The model under review builds one solid part; all positions refer to its coordinate system, in mm. A direction names the side the tool comes from. Round coordinates to 2 decimals unless told otherwise and drop trailing zeros. Write each loop counter-clockwise with the first axis right and the second up, starting at its lowest first coordinate (ties: lowest second). Pieces come first, ordered by that corner, then holes. Notation, with made-up numbers: (31, 69.5) -> (57, 69.5) arc R24 cw to (57, 84.5) -> close; hole circle Ø11 at (38.25, -35). An arc over 180 degrees is marked (long way). Use CSV: the item, a comma, the result in double quotes. Start each with the question number.
1) Take a section at C-C, the plane z = 3.5. Give the boundary of the cut face in (x, y).
2) Mouldability with a two-part tool opening along X and no side actions: class faces 4 (the face through (21.4, -0.1, 0.5)), 5 (the face through (-21.4, -0.1, 0.5)), 6 (the face through (-13, -0.76, 6.28)), 7 (the face through (-20.45, 8.5, 0.51)) as released by +X, released by -X, zero draft, split by the parting line, or undercut.
3) Take a section at B-B, the plane x = 15.4. Give the boundary of the cut face in (y, z), then the cut area to 3 significant figures.
4) Take a section at A-A, the plane y = 7.5. Give the boundary of the cut face in (x, z).
5) Machinability: for faces 1 (the face through (11.7, 7, 6)), 2 (the face through (0.55, -3, 6)), 3 (the face through (7, 5.25, 6)), which of the approach directions +Z, -Z, +X, -X, +Y, -Y give a long, thin tool a straight path to every point of the face, cutting with its end or side? Answer none if there is none.
6) For pin 1 Ø4.5 at (y, z) = (8.5, 6.5) entering from +X; pin 2 Ø3 at (y, z) = (-7.5, 8) entering from +X; pin 3 Ø5.5 at (x, z) = (3.5, 5.5) entering from -Y; pin 4 Ø2.5 at (x, y) = (15.4, -8.5) entering from +Z, all flat-tipped, find the tip position at first contact; note any pin that passes through.
7) Wall thickness on probe 1 along Y at (x, z) = (-20.05, 0.25); probe 2 along Y at (x, z) = (8.5, 10.25); probe 3 along Z at (x, y) = (-19, 8): over which ranges is each line inside the solid? List them lowest first. Write a range as [from, to].
8) Take a section at D-D, the plane y = 0.75. Give the boundary of the cut face in (x, z).
from build123d import *

# Parameters (mm, degrees)
SKETCH1_W           = 42.8
SKETCH1_H           = 20.5
SKETCH1_R           = 1.4
BOSS_EXTRUDE1_DEPTH = 1
SKETCH3_R           = 3.95
SKETCH3_W           = 9.3
SKETCH3_H           = 4.3
SKETCH3_W_2         = 12.05
SKETCH3_H_2         = 12.05
BOSS_EXTRUDE2_DEPTH = 10.7
SKETCH4_R           = 0.5
CUT_EXTRUDE1_DEPTH  = 2


with BuildPart() as part:
    # Sketch1 → Boss-Extrude1 (new body)
    with BuildSketch(Plane.XY):
        Rectangle(SKETCH1_W, SKETCH1_H)
        with Locations((15.4, -8.5)):
            Circle(SKETCH1_R, mode=Mode.SUBTRACT)
        with Locations((-15.4, 8.5)):
            Circle(SKETCH1_R, mode=Mode.SUBTRACT)
    extrude(amount=BOSS_EXTRUDE1_DEPTH)

    # Sketch3 → Boss-Extrude2 (add)
    with BuildSketch(Plane.XY.offset(1)):
        with Locations((16.65, 0.75)):
            Circle(SKETCH3_R)
        with Locations((-16.65, 0.75)):
            Circle(SKETCH3_R)
        with Locations((7.05, 7.4)):
            Rectangle(SKETCH3_W, SKETCH3_H)
        with Locations((6.575, -2.575)):
            Rectangle(SKETCH3_W_2, SKETCH3_H_2)
    extrude(amount=BOSS_EXTRUDE2_DEPTH)

    # Sketch4 → Cut-Extrude1 (cut, through all)
    with BuildSketch(Plane.XY.offset(1)):
        with Locations((-20.05, 8.8)):
            Circle(SKETCH4_R)
        with Locations((-20.05, -8.8)):
            Circle(SKETCH4_R)
        with Locations((20.05, -8.8)):
            Circle(SKETCH4_R)
        with Locations((20.05, 8.8)):
            Circle(SKETCH4_R)
    extrude(amount=-CUT_EXTRUDE1_DEPTH, mode=Mode.SUBTRACT)


solid = part.part
Values found:
1,outline,"circle Ø7.9 at (-16.65, 0.75); (0.55, -8.6) -> (12.6, -8.6) -> (12.6, 3.45) -> (0.55, 3.45) -> close; (2.4, 5.25) -> (11.7, 5.25) -> (11.7, 9.55) -> (2.4, 9.55) -> close; circle Ø7.9 at (16.65, 0.75)"
2,face 4,"released by +X"
2,face 5,"released by -X"
2,face 6,"undercut"
2,face 7,"undercut"
3,outline,"(-10.25, 0) -> (-9.9, 0) -> (-9.9, 1) -> (-10.25, 1) -> close; (-7.1, 0) -> (10.25, 0) -> (10.25, 1) -> (4.5, 1) -> (4.5, 11.7) -> (-3, 11.7) -> (-3, 1) -> (-7.1, 1) -> close"
3,area,"97.9 mm²"
4,outline,"(-21.4, 0) -> (-16.38, 0) -> (-16.38, 1) -> (-21.4, 1) -> close; (-14.42, 0) -> (21.4, 0) -> (21.4, 1) -> (11.7, 1) -> (11.7, 11.7) -> (2.4, 11.7) -> (2.4, 1) -> (-14.42, 1) -> close"
5,face 1,"+Z, +X, +Y"
5,face 2,"+Z, +Y, -Y"
5,face 3,"+Z, +X, -X"
6,pin 1,"x = 11.7"
6,pin 2,"x = 12.6"
6,pin 3,"y = -8.6"
6,pin 4,"through"
7,probe 1,"[-10.25, -9.3], [-8.3, 8.3], [9.3, 10.25]"
7,probe 2,"[-8.6, 3.45], [5.25, 9.55]"
7,probe 3,"[0, 1]"
8,outline,"(-21.4, 0) -> (21.4, 0) -> (21.4, 1) -> (20.6, 1) -> (20.6, 11.7) -> (12.7, 11.7) -> (12.7, 1) -> (12.6, 1) -> (12.6, 11.7) -> (0.55, 11.7) -> (0.55, 1) -> (-12.7, 1) -> (-12.7, 11.7) -> (-20.6, 11.7) -> (-20.6, 1) -> (-21.4, 1) -> close"
